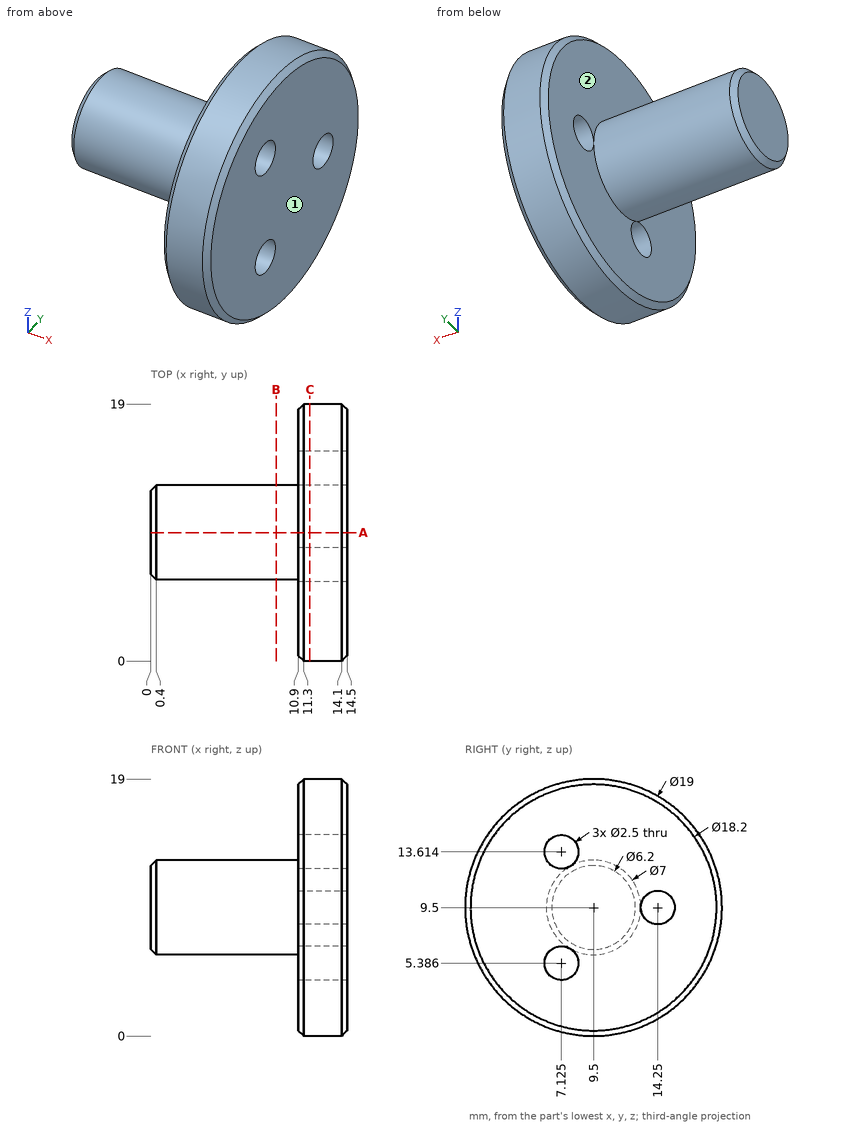
Source: three-view drawing plus pictorial views. Frame: mm from the lowest corner of the part. A direction names the side the tool comes from. Coordinates: 2 decimals unless noted, no trailing zeros. Write each loop counter-clockwise with the first axis right and the second up, starting at its lowest first coordinate (ties: lowest second). Pieces come first, ordered by that corner, then holes. Notation, with made-up numbers: (47.5, 62) - (92.5, 62) arc R26 ccw to (92.5, 88) - close; hole circle Ø3 at (88, 54). An arc over 180 degrees is marked (long way). Return JSON: item names as keys, results as strings.
Item 1: Section query B-B (x = 9.25). Output: boundary loops of the cut face in (y, z), and give its area (3 significant figures).
Completed:
{"outline": "circle Ø7 at (9.5, 9.5)", "area": "38.5 mm2"}
Item 2: Section query C-C (x = 11.75). Count the separate pieces of the cut face and the enclosed holes in it, and give its area (3 significant figures).
Completed:
{"separate pieces": "1", "enclosed holes": "3", "area": "269 mm2"}
Item 3: Pin query (flat end, axial travel): pin 1 Ø4 at (y, z) = (7.13, 13.61) entering from -X; pin 2 Ø3 at (x, y) = (10, 14.5) entering from -Z (1 decimal); pin 3 Ø1.5 at (x, z) = (12, 5.5) entering from -Y. Return the tip coordinate at first contact, or that it passes through.
Completed:
{"pin 1": "stops at x = 0", "pin 2": "stops at z = 1", "pin 3": "stops at y = 0.57"}
Item 4: Section query A-A (y = 9.5). Output: boundary loops of the cut face in (x, z).
Completed:
{"outline": "(0, 6.4) - (0.4, 6) - (10.9, 6) - (10.9, 0.4) - (11.3, 0) - (14.1, 0) - (14.5, 0.4) - (14.5, 18.6) - (14.1, 19) - (11.3, 19) - (10.9, 18.6) - (10.9, 13) - (0.4, 13) - (0, 12.6) - close"}
Item 5: Line query: L1, parallel to Y at x = 13.4, z = 9.5; L2, parallel to X at y = 17.25, z = 13.5; L3, parallel to Y at x = 13.75, z = 1.5 (1 decimal). Output: solid intervals per line, ascending.
Completed:
{"L1": "y = 0 to 13, 15.5 to 19", "L2": "x = 10.9 to 14.5", "L3": "y = 4.4 to 14.6"}
Item 6: Reachability of the marked faces 1 and 2 from +Z, -Z, +X, -X, +Y, -Y: full face, straight path, thin tool, end or side. Return the list, or none.
Completed:
{"face 1": "+Z, -Z, +X, +Y, -Y", "face 2": "-X"}
